Check sheet for the modelled part. Datum: model origin and axes. Units: mm. Give positions to 0.01 mm unless a question says otherwise; leave off trailing zeros. Order: outer loops, then holes, each group sorted by start corner. A loop starts at its lowest first (then second) coordinate and runs counter-clockwise, first axis right, second up.
```python
from build123d import *

# Parameters (mm, degrees)
EXTRUSION1_DEPTH        = 150
PER_AGE1_OUTLINE_R      = 2.1
PER_AGE1_DEPTH          = 150
ENL_V_MAT_EXTRU_1_DEPTH = 300
ENL_V_MAT_EXTRU_3_DEPTH = 300
ENL_V_MAT_EXTRU_4_DEPTH = 151.665191733
ENL_V_MAT_EXTRU_7_DEPTH = 151.665191733


# Read off the part's stored shape, not the designer's step: Perçage1
with BuildPart() as part:
    # Esquisse1 → Extrusion1 (new body)
    with BuildSketch(Plane.XY):
        with BuildLine():
            Line((-10, 8), (-10, -8))
            ThreePointArc((-10, -8), (-9.414213562, -9.414213562), (-8, -10))
            Line((-8, -10), (8, -10))
            ThreePointArc((8, -10), (9.414213562, -9.414213562), (10, -8))
            Line((10, -8), (10, 8))
            ThreePointArc((10, 8), (9.414213562, 9.414213562), (8, 10))
            Line((8, 10), (-8, 10))
            ThreePointArc((-8, 10), (-9.414213562, 9.414213562), (-10, 8))
        make_face()
    extrude(amount=EXTRUSION1_DEPTH)

    # Perçage1 outline → Perçage1 (cut)
    with BuildSketch(Plane.XY):
        Circle(PER_AGE1_OUTLINE_R)
    extrude(amount=PER_AGE1_DEPTH, mode=Mode.SUBTRACT)

    # Esquisse3 → Enlèv. mat.-Extru.1 (cut)
    with BuildSketch(Plane.XY.offset(150)):
        Polygon((10, 2.5), (8.2, 2.5), (8.2, 6), (3.7, 2.5), (3.7, -2.5), (8.2, -6), (8.2, -2.5), (10, -2.5), align=None)
    extrude(amount=-ENL_V_MAT_EXTRU_1_DEPTH, mode=Mode.SUBTRACT)

    # Esquisse5 → Enlèv. mat.-Extru.3 (cut)
    with BuildSketch(Plane.XY.offset(150)):
        Polygon((-2.5, 10), (-2.5, 8.2), (-6, 8.2), (-2.5, 3.7), (2.5, 3.7), (6, 8.2), (2.5, 8.2), (2.5, 10), align=None)
    extrude(amount=-ENL_V_MAT_EXTRU_3_DEPTH, mode=Mode.SUBTRACT)

    # Esquisse6 → Enlèv. mat.-Extru.4 (cut, through all)
    with BuildSketch(Plane.XY.offset(150)):
        Polygon((-2.5, -10), (-2.5, -8.2), (-6, -8.2), (-2.5, -3.7), (2.5, -3.7), (6, -8.2), (2.5, -8.2), (2.5, -10), align=None)
    extrude(amount=-ENL_V_MAT_EXTRU_4_DEPTH, mode=Mode.SUBTRACT)

    # Esquisse4 → Enlèv. mat.-Extru.7 (cut, through all)
    with BuildSketch(Plane.XY.offset(150)):
        Polygon((-10, 2.5), (-8.2, 2.5), (-8.2, 6), (-3.7, 2.5), (-3.7, -2.5), (-8.2, -6), (-8.2, -2.5), (-10, -2.5), align=None)
    extrude(amount=-ENL_V_MAT_EXTRU_7_DEPTH, mode=Mode.SUBTRACT)


solid = part.part
```
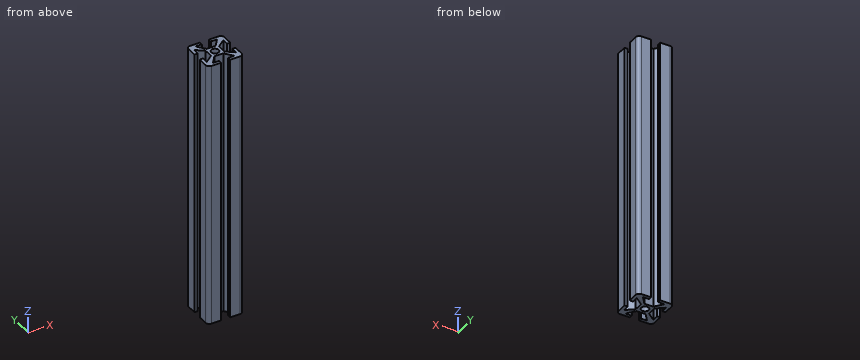
(1) Material ranges on L1, parallel to Y at x = 0, z = 89; L2, parallel to Y at x = -4, z = 82.5; L3, parallel to X at y = 2.75, z = 48.5, recorded low to high.
Response values:
L1: y = -3.7 to -2.1, 2.1 to 3.7
L2: y = -10 to -8.2, -5.63 to -2.73, 2.73 to 5.63, 8.2 to 10
L3: x = -10 to -8.2, -4.02 to 4.02, 8.2 to 10
(2) Cross-section at A-A on x = 0. Enter the section's corners in (y, z).
Response values:
outline: (-3.7, 0) - (-2.1, 0) - (-2.1, 150) - (-3.7, 150) - close; (2.1, 0) - (3.7, 0) - (3.7, 150) - (2.1, 150) - close
(3) Gauge pin test, flat ends, axial feed: pin 1 Ø0.5 at (y, z) = (9, 109.5) entering from -X; pin 2 Ø1.4 at (x, z) = (-9, 111.5) entering from -Y; pin 3 Ø3 at (y, z) = (-0.5, 24) entering from -X; pin 4 Ø5.5 at (x, z) = (1, 44.5) entering from +Y. Record the tip position at first contact, or that the pin passes through.
Response values:
pin 1: stops at x = -9.85
pin 2: stops at y = -9.98
pin 3: stops at x = -3.7
pin 4: stops at y = 10
